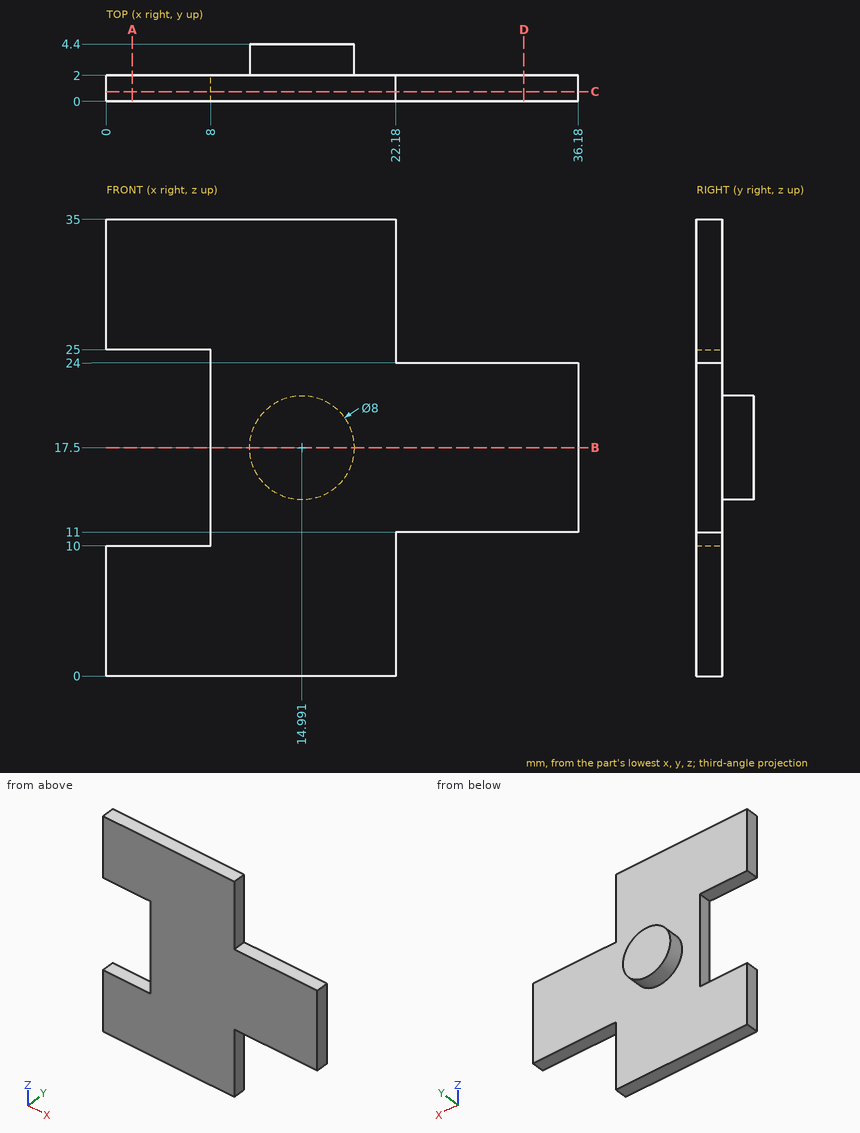
Check sheet for the drawn part. Datum: minimum x, y, z corner. Units: mm. Coordinates: 2 decimals unless noted, no trailing zeros. Write each loop counter-clockwise with the first axis right and the second up, starting at its lowest first coordinate (ties: lowest second). Pieces come first, ordered by that corner, then holes. Notation, with made-up numbers: M 87,53.25 L 122,53.25 A30 cw 122,82.25 Z; hole C 41.25,17.25 d6. An arc over 180 degrees is marked long. One line per item, written item: value.
Item 1: Gauge pin test, flat ends, axial feed: pin 1 Ø1 at (y, z) = (1, 3) entering from +X; pin 2 Ø6 at (x, z) = (6.5, 17) entering from +Y; pin 3 Ø1 at (x, y) = (29, 0.5) entering from +Z. Record the tip position at first contact, or that the pin passes through.
Check sheet entries:
pin 1: stops at x = 22.18
pin 2: stops at y = 2
pin 3: stops at z = 24
Item 2: Section check A-A, the plane x = 2. Record the boundary of the cut face in (y, z).
Check sheet entries:
outline: M 0,0 L 2,0 L 2,10 L 0,10 Z; M 0,25 L 2,25 L 2,35 L 0,35 Z
Item 3: Section check B-B, the plane z = 17.5. Record the boundary of the cut face in (x, y).
Check sheet entries:
outline: M 8,0 L 36.18,0 L 36.18,2 L 18.99,2 L 18.99,4.4 L 10.99,4.4 L 10.99,2 L 8,2 Z
Item 4: Section check D-D, the plane x = 32. Record the boundary of the cut face in (y, z).
Check sheet entries:
outline: M 0,11 L 2,11 L 2,24 L 0,24 Z
Item 5: Section check C-C, the plane y = 0.75. Record the boundary of the cut face in (x, z), plus the area to 3 significant figures.
Check sheet entries:
outline: M 0,0 L 22.18,0 L 22.18,11 L 36.18,11 L 36.18,24 L 22.18,24 L 22.18,35 L 0,35 L 0,25 L 8,25 L 8,10 L 0,10 Z
area: 838 mm^2
Item 6: Scan lines: line 1 along X through (y, z) = (0.3, 10.5); line 2 along Y through (x, z) = (29, 18); line 3 along X through (y, z) = (1.05, 27.5). Record each from-to range of solid material in increasing order.
Check sheet entries:
line 1: x = 8 to 22.18
line 2: y = 0 to 2
line 3: x = 0 to 22.18
